Read the model definition and answer for the solid it produces. Units are mm, in the model's axes. Coordinates: 2 decimals unless noted, no trailing zeros. Write each loop counter-clockwise with the first axis right and the second up, starting at its lowest first coordinate (ties: lowest second). Pieces come first, ordered by that corner, then holes. Notation, with made-up numbers: (30.25, 84.25) -> (86.25, 84.25) arc R15 ccw to (86.25, 99.25) -> close; hole circle Ø9 at (-17.5, 19.5). An arc over 180 degrees is marked (long way). One line per item, written item: value. Start each with the question number.
1. Find section A-A, the plane x = -7. Write down the section's boundary in (y, z), and give its area (3 significant figures).
2. Find section C-C, the plane z = 6.25. Write down the section's boundary in (x, y).
3. Consider line 1 along Z through (x, y) = (3, 7); line 2 along Y through (x, z) = (5.25, 6.75); line 3 along Y through (x, z) = (-4, 5.5). Determine where each line is inside the solid, lowest interval first.
4. Find section B-B, the plane y = 6.75. Write down the section's boundary in (x, z).
```python
from build123d import *

# Parameters (mm, degrees)
ESQUISSE1_W        = 15.52
ESQUISSE1_H        = 15.52
BOSS_EXTRU_1_DEPTH = 7.76
CONG_1_R           = 3


with BuildPart() as part:
    # Esquisse1 → Boss.-Extru.1 (new body)
    with BuildSketch(Plane.XY):
        Rectangle(ESQUISSE1_W, ESQUISSE1_H)
    extrude(amount=BOSS_EXTRU_1_DEPTH)

    # Congé1
    cong_1_edges = [part.edges().sort_by_distance(p)[0] for p in [
        (0, 7.76, 7.76),
    ]]
    fillet(cong_1_edges, radius=CONG_1_R)


solid = part.part
```
Answer block:
1. outline: (-7.76, 0) -> (7.76, 0) -> (7.76, 4.76) arc R3 ccw to (4.76, 7.76) -> (-7.76, 7.76) -> close
1. area: 119 mm2
2. outline: (-7.76, -7.76) -> (7.76, -7.76) -> (7.76, 7.36) -> (-7.76, 7.36) -> close
3. line 1: z = 0 to 6.76
3. line 2: y = -7.76 to 7
3. line 3: y = -7.76 to 7.67
4. outline: (-7.76, 0) -> (7.76, 0) -> (7.76, 7) -> (-7.76, 7) -> close
